Input: part model. Units: mm. Frame: model coordinates. Coordinates: 2 decimals unless noted, no trailing zeros. Loops run counter-clockwise (first coordinate to the right, second up) from the corner with the lowest first, then second, coordinate; pieces in that order, holes last.
Item 1: Section A-A on z = 0. Return loops of the section in (x, y), and give its area (3 significant figures).
Item 2: Ray query, line 1 along X through (y, z) = (4.3, -0.5); line 2 along X through (y, z) = (2.1, -1); line 3 along Z through (x, y) = (166, 0.8). Return the intervals inside material, ascending.
Item 3: Section B-B on y = 3.3. Return loops of the section in (x, z).
Item 4: Section C-C on x = 112. Return loops of the section in (y, z), and give its area (3 significant figures).
```python
from build123d import *

# Parameters (mm, degrees)
SKETCH_1_W          = 620
SKETCH_1_H          = 30
EXTRUDE_1_DEPTH     = 6
CUT_EXTRUDE_1_DEPTH = 311.420682301


with BuildPart() as part:
    # 草图1 → 凸台-拉伸1 (new body)
    with BuildSketch(Plane(origin=(0, 0, 0), x_dir=(1, 0, 0), z_dir=(0, 1, 0))):
        Rectangle(SKETCH_1_W, SKETCH_1_H)
    extrude(amount=EXTRUDE_1_DEPTH)

    # 草图2 → 切除-拉伸1 (cut, through all)
    with BuildSketch(Plane(origin=(0, 6, 0), x_dir=(1, 0, 0), z_dir=(0, 1, 0))):
        with BuildLine():
            Line((30, -7.5), (-30, -7.5))
            ThreePointArc((-30, -7.5), (-37.5, 0), (-30, 7.5))
            Line((-30, 7.5), (30, 7.5))
            ThreePointArc((30, 7.5), (37.5, 0), (30, -7.5))
        make_face()
        with BuildLine():
            Line((-60, -7.5), (-180, -7.5))
            ThreePointArc((-180, -7.5), (-187.5, 0), (-180, 7.5))
            Line((-180, 7.5), (-60, 7.5))
            ThreePointArc((-60, 7.5), (-52.5, 0), (-60, -7.5))
        make_face()
        with BuildLine():
            Line((60, 7.5), (180, 7.5))
            ThreePointArc((180, 7.5), (187.5, 0), (180, -7.5))
            Line((180, -7.5), (60, -7.5))
            ThreePointArc((60, -7.5), (52.5, 0), (60, 7.5))
        make_face()
    extrude(amount=-CUT_EXTRUDE_1_DEPTH, mode=Mode.SUBTRACT)


solid = part.part
```
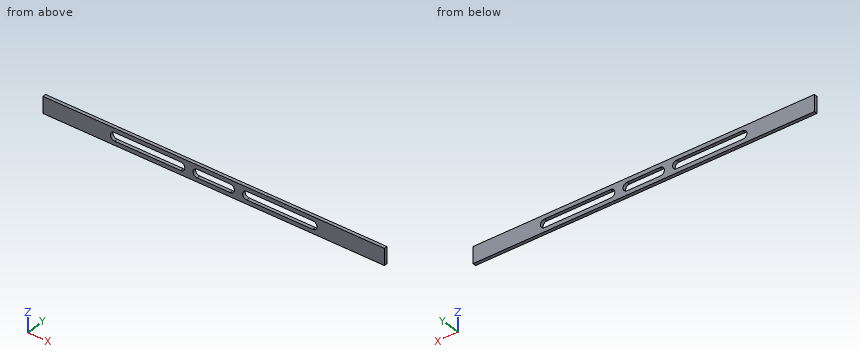
Results found:
1. outline: (-310, 0) - (-187.5, 0) - (-187.5, 6) - (-310, 6) - close; (-52.5, 0) - (-37.5, 0) - (-37.5, 6) - (-52.5, 6) - close; (37.5, 0) - (52.5, 0) - (52.5, 6) - (37.5, 6) - close; (187.5, 0) - (310, 0) - (310, 6) - (187.5, 6) - close
1. area: 1,650 mm2
2. line 1: x = -310 to -187.48, -52.52 to -37.48, 37.48 to 52.52, 187.48 to 310
2. line 2: x = -310 to -187.43, -52.57 to -37.43, 37.43 to 52.57, 187.43 to 310
2. line 3: z = -15 to -7.5, 7.5 to 15
3. outline: (-310, -15) - (310, -15) - (310, 15) - (-310, 15) - close; hole (-180, -7.5) - (-60, -7.5) arc R7.5 ccw to (-60, 7.5) - (-180, 7.5) arc R7.5 ccw to start; hole (-30, -7.5) - (30, -7.5) arc R7.5 ccw to (30, 7.5) - (-30, 7.5) arc R7.5 ccw to start; hole (60, -7.5) - (180, -7.5) arc R7.5 ccw to (180, 7.5) - (60, 7.5) arc R7.5 ccw to start
4. outline: (0, -15) - (6, -15) - (6, -7.5) - (0, -7.5) - close; (0, 7.5) - (6, 7.5) - (6, 15) - (0, 15) - close
4. area: 90.0 mm2
